Can you work these out from the model? Positions are in its coordinate system, mm. Give positions to 0.01 mm unless a question says otherwise; leave off trailing zeros.
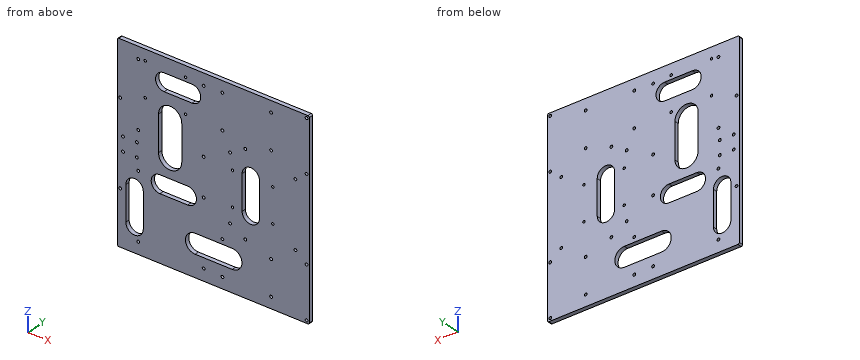
```python
from build123d import *

# Parameters (mm, degrees)
SKETCH_1_W              = 276
SKETCH_1_H              = 276
EXTRUDE_1_DEPTH         = 6
FILLET_1_R              = 2
SKETCH_2_R              = 2
CUT_EXTRUDE_1_DEPTH     = 6
SKETCH_10_R             = 2
CUT_EXTRUDE_1980_DEPTH  = 7
SKETCH_4_R              = 2
CUT_EXTRUDE_94_94_DEPTH = 6
SKETCH_8_R              = 1.75
RPI4_DEPTH              = 6
CUT_EXTRUDE_5_DEPTH     = 6


with BuildPart() as part:
    # Sketch 1 → Extrude 1 (new body)
    with BuildSketch(Plane(origin=(0, 0, 0), x_dir=(1, 0, 0), z_dir=(0, 1, 0))):
        Rectangle(SKETCH_1_W, SKETCH_1_H)
    extrude(amount=EXTRUDE_1_DEPTH)

    # Fillet 1
    fillet_1_edges = [part.edges().sort_by_distance(p)[0] for p in [
        (138, 3, 138),
        (-138, 3, 138),
        (-138, 3, -138),
        (138, 3, -138),
    ]]
    fillet(fillet_1_edges, radius=FILLET_1_R)

    # Sketch 2 → Cut-Extrude 1 (cut)
    with BuildSketch(Plane(origin=(0, 6, 0), x_dir=(1, 0, 0), z_dir=(0, 1, 0))):
        with Locations(Location((-134, 60, 0), (0, 0, 270))):
            Circle(SKETCH_2_R)
        with Locations(Location((134, 60, 0), (0, 0, 90))):
            Circle(SKETCH_2_R)
        with Locations(Location((134, -60, 0), (0, 0, 270))):
            Circle(SKETCH_2_R)
        with Locations(Location((-134, -60, 0), (0, 0, 90))):
            Circle(SKETCH_2_R)
        with Locations(Location((46, 60, 0), (0, 0, 270))):
            Circle(SKETCH_2_R)
        with Locations(Location((46, -60, 0), (0, 0, 90))):
            Circle(SKETCH_2_R)
        with Locations(Location((134, 134, 0), (0, 0, 270))):
            Circle(SKETCH_2_R)
        with Locations(Location((134, -134, 0), (0, 0, 90))):
            Circle(SKETCH_2_R)
    extrude(amount=-CUT_EXTRUDE_1_DEPTH, mode=Mode.SUBTRACT)

    # Sketch 10 → Cut-Extrude 1980 (cut)
    with BuildSketch(Plane(origin=(0, 6, 0), x_dir=(1, 0, 0), z_dir=(0, 1, 0))):
        with Locations(Location((13, 122, 0), (0, 0, 270))):
            Circle(SKETCH_10_R)
        with Locations(Location((83, 122, 0), (0, 0, 90))):
            Circle(SKETCH_10_R)
        with Locations(Location((13, 72, 0), (0, 0, 90))):
            Circle(SKETCH_10_R)
        with Locations(Location((83, 72, 0), (0, 0, 270))):
            Circle(SKETCH_10_R)
        with Locations(Location((-130, 10, 0), (0, 0, 270))):
            Circle(SKETCH_10_R)
        with Locations(Location((-110, 10, 0), (0, 0, 270))):
            Circle(SKETCH_10_R)
        with Locations(Location((-110, -10, 0), (0, 0, 270))):
            Circle(SKETCH_10_R)
        with Locations(Location((-130, -10, 0), (0, 0, 270))):
            Circle(SKETCH_10_R)
        with Locations(Location((83, -72, 0), (0, 0, 90))):
            Circle(SKETCH_10_R)
        with Locations(Location((13, -72, 0), (0, 0, 270))):
            Circle(SKETCH_10_R)
        with Locations(Location((83, -122, 0), (0, 0, 270))):
            Circle(SKETCH_10_R)
        with Locations(Location((13, -122, 0), (0, 0, 90))):
            Circle(SKETCH_10_R)
    extrude(amount=-CUT_EXTRUDE_1980_DEPTH, mode=Mode.SUBTRACT)

    # Sketch 4 → Cut-Extrude 94_94 (cut)
    with BuildSketch(Plane(origin=(0, 6, 0), x_dir=(1, 0, 0), z_dir=(0, 1, 0))):
        with Locations(Location((-108, 121, 0), (0, 0, 270))):
            Circle(SKETCH_4_R)
        with Locations(Location((-14, 121, 0), (0, 0, 270))):
            Circle(SKETCH_4_R)
        with Locations(Location((-14, 27, 0), (0, 0, 90))):
            Circle(SKETCH_4_R)
        with Locations(Location((-108, 27, 0), (0, 0, 90))):
            Circle(SKETCH_4_R)
        with Locations(Location((-108, -27, 0), (0, 0, 270))):
            Circle(SKETCH_4_R)
        with Locations(Location((-14, -27, 0), (0, 0, 270))):
            Circle(SKETCH_4_R)
        with Locations(Location((-14, -121, 0), (0, 0, 90))):
            Circle(SKETCH_4_R)
        with Locations(Location((-108, -121, 0), (0, 0, 90))):
            Circle(SKETCH_4_R)
        with Locations(Location((24, 47, 0), (0, 0, 270))):
            Circle(SKETCH_4_R)
        with Locations(Location((118, 47, 0), (0, 0, 270))):
            Circle(SKETCH_4_R)
        with Locations(Location((118, -47, 0), (0, 0, 90))):
            Circle(SKETCH_4_R)
        with Locations(Location((24, -47, 0), (0, 0, 90))):
            Circle(SKETCH_4_R)
    extrude(amount=-CUT_EXTRUDE_94_94_DEPTH, mode=Mode.SUBTRACT)

    # Sketch 8 → RPi4 (cut)
    with BuildSketch(Plane(origin=(0, 6, 0), x_dir=(1, 0, 0), z_dir=(0, 1, 0))):
        with Locations(Location((85.46549702, 24.5, 0), (0, 0, 270))):
            Circle(SKETCH_8_R)
        with Locations(Location((27.46549702, 24.5, 0), (0, 0, 270))):
            Circle(SKETCH_8_R)
        with Locations(Location((27.46549702, -24.5, 0), (0, 0, 270))):
            Circle(SKETCH_8_R)
        with Locations(Location((85.46549702, -24.5, 0), (0, 0, 270))):
            Circle(SKETCH_8_R)
        with Locations(Location((-40, -73.5, 0), (0, 0, 270))):
            Circle(SKETCH_8_R)
        with Locations(Location((-98, -73.5, 0), (0, 0, 270))):
            Circle(SKETCH_8_R)
        with Locations(Location((-98, -122.5, 0), (0, 0, 270))):
            Circle(SKETCH_8_R)
        with Locations(Location((-40, -122.5, 0), (0, 0, 270))):
            Circle(SKETCH_8_R)
    extrude(amount=-RPI4_DEPTH, mode=Mode.SUBTRACT)

    # Sketch 6 → Cut-Extrude 5 (cut)
    with BuildSketch(Plane(origin=(0, 6, 0), x_dir=(1, 0, 0), z_dir=(0, 1, 0))):
        with BuildLine():
            Line((-70.62792666, -91.796358409), (-30.62792666, -91.796358409))
            ThreePointArc((-30.62792666, -91.796358409), (-18.12792666, -104.296358409), (-30.62792666, -116.796358409))
            Line((-30.62792666, -116.796358409), (-70.62792666, -116.796358409))
            ThreePointArc((-70.62792666, -116.796358409), (-83.12792666, -104.296358409), (-70.62792666, -91.796358409))
        make_face()
        with BuildLine():
            Line((-76.854148501, 45.577500198), (-36.854148501, 45.577500198))
            ThreePointArc((-36.854148501, 45.577500198), (-24.354148501, 33.077500198), (-36.854148501, 20.577500198))
            Line((-36.854148501, 20.577500198), (-76.854148501, 20.577500198))
            ThreePointArc((-76.854148501, 20.577500198), (-89.354148501, 33.077500198), (-76.854148501, 45.577500198))
        make_face()
        with BuildLine():
            Line((-125.792186218, 101.779020019), (-125.792186218, 51.779020019))
            ThreePointArc((-125.792186218, 51.779020019), (-113.292186218, 39.279020019), (-100.792186218, 51.779020019))
            Line((-100.792186218, 51.779020019), (-100.792186218, 101.779020019))
            ThreePointArc((-100.792186218, 101.779020019), (-113.292186218, 114.279020019), (-125.792186218, 101.779020019))
        make_face()
        with BuildLine():
            Line((-26.207579038, 106.773909834), (27.18238493, 106.773909834))
            ThreePointArc((27.18238493, 106.773909834), (41.090694872, 92.865599892), (27.18238493, 78.957289951))
            Line((27.18238493, 78.957289951), (-26.207579038, 78.957289951))
            ThreePointArc((-26.207579038, 78.957289951), (-40.115888979, 92.865599892), (-26.207579038, 106.773909834))
        make_face()
        with BuildLine():
            Line((-78.86378902, -7.888425697), (-78.86378902, -59.108123383))
            ThreePointArc((-78.86378902, -59.108123383), (-62.147948764, -75.823963639), (-45.432108508, -59.108123383))
            Line((-45.432108508, -59.108123383), (-45.432108508, -7.888425697))
            ThreePointArc((-45.432108508, -7.888425697), (-62.147948764, 8.827414559), (-78.86378902, -7.888425697))
        make_face()
        with BuildLine():
            Line((41.348697743, 24.533398762), (41.348697743, -25.466601238))
            ThreePointArc((41.348697743, -25.466601238), (53.848697743, -37.966601238), (66.348697743, -25.466601238))
            Line((66.348697743, -25.466601238), (66.348697743, 24.533398762))
            ThreePointArc((66.348697743, 24.533398762), (53.848697743, 37.033398762), (41.348697743, 24.533398762))
        make_face()
    extrude(amount=-CUT_EXTRUDE_5_DEPTH, mode=Mode.SUBTRACT)


solid = part.part
```
1) Please list where these lines run through material, in increasing order: L1, parallel to X at y = 5.45, z = -51.5; L2, parallel to Z at x = -1.5, y = 4.45; L3, parallel to X at y = 5.7, z = 23.
Values follow:
L1: x = -138 to -125.79, -100.8 to 138
L2: z = -138 to -106.77, -78.96 to 138
L3: x = -138 to -78.86, -45.43 to 26.56, 28.37 to 41.35, 66.35 to 84.56, 86.37 to 138
2) For pin 1 Ø2.5 at (x, z) = (134, 134) entering from -Y, with a flat end and sliding along its axis, tell me the tip position at first contact or that it passes through.
Values follow:
pin 1: passes through
3) Suppose I cut it at A-A on y = 2.4. State how many separate pieces and enclosed holes the cut face has, plus the area to 3 significant figures.
Values follow:
separate pieces: 1
enclosed holes: 46
area: 64,500 mm2
